The figure shows three views and two pictorial views of one solid part (mm, origin at its lowest corner). Answer the questions. Give positions to 0.01 mm unless a question says otherwise; leave off trailing zeros. Loops run counter-clockwise (first coordinate to the right, second up) from the corner with the lowest first, then second, coordinate; pieces in that order, holes last. Notation, with made-up numbers: (37, 37.5) -> (77, 37.5) arc R24 cw to (77, 51.5) -> close; hole circle Ø5 at (36, -17). An arc over 180 degrees is marked (long way). Answer as CSV lines item,"result". Start each with the question number.
1. Find section C-C, the plane y = 81. Give the vertices of the cut face in (x, z), and give its area (3 significant figures).
2. Flat-ended cylindrical pins translate along their axes: pin 1 Ø3.5 at (x, y) = (11, 152) entering from -Z; pin 2 Ø0.9 at (x, z) = (79.5, 5) entering from +Y; pin 3 Ø1.5 at (x, z) = (80, 5) entering from -Y. Find the tip coordinate at first contact, or state that the pin passes through.
3. Find the intervals of material crossed by line 1 along X through (y, z) = (72, 12.5); line 2 along Y through (x, z) = (29, 8.5); line 3 along Y through (x, z) = (72.5, 6.5), in increasing order.
4. Find section A-A, the plane x = 71. Give the vertices of the cut face in (y, z).
5. Find section B-B, the plane y = 13. Give the vertices of the cut face in (x, z).
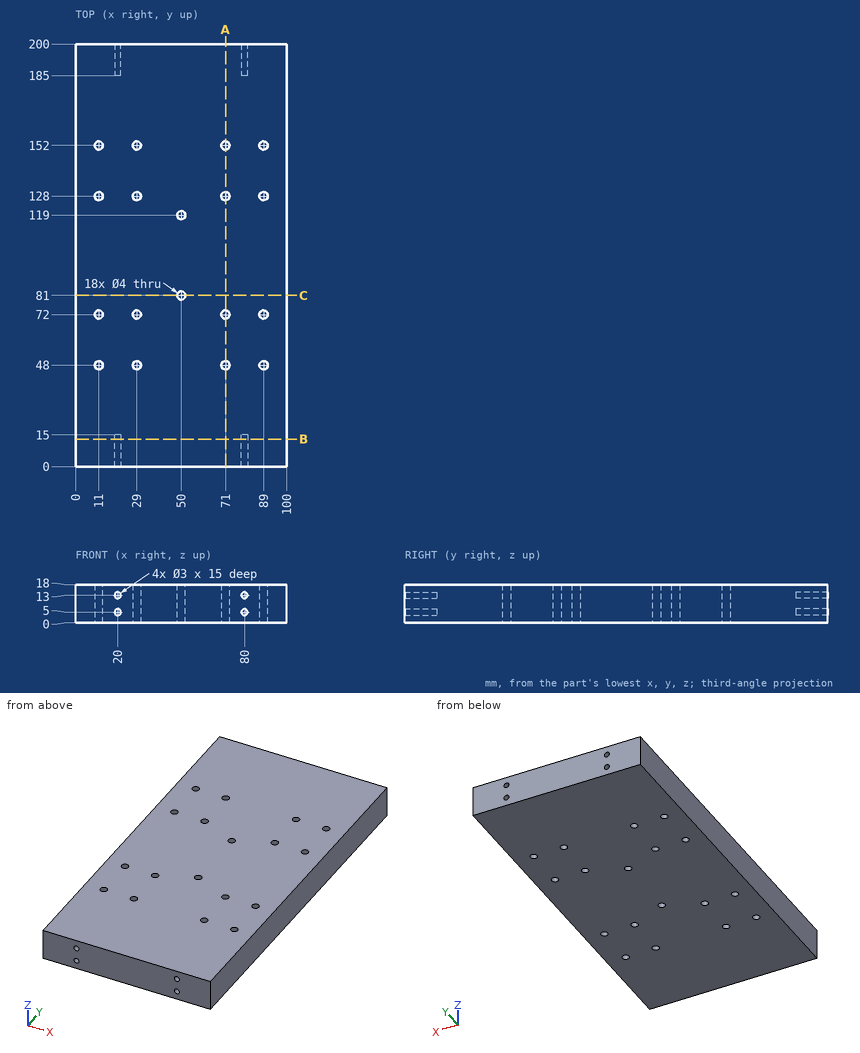
Resolved:
1,outline,"(0, 0) -> (48, 0) -> (48, 18) -> (0, 18) -> close; (52, 0) -> (100, 0) -> (100, 18) -> (52, 18) -> close"
1,area,"1,730 mm^2"
2,pin 1,"passes through"
2,pin 2,"stops at y = 185"
2,pin 3,"stops at y = 15"
3,line 1,"x = 0 to 9, 13 to 27, 31 to 69, 73 to 87, 91 to 100"
3,line 2,"y = 0 to 46, 50 to 70, 74 to 126, 130 to 150, 154 to 200"
3,line 3,"y = 0 to 46.68, 49.32 to 70.68, 73.32 to 126.68, 129.32 to 150.68, 153.32 to 200"
4,outline,"(0, 0) -> (46, 0) -> (46, 18) -> (0, 18) -> close; (50, 0) -> (70, 0) -> (70, 18) -> (50, 18) -> close; (74, 0) -> (126, 0) -> (126, 18) -> (74, 18) -> close; (130, 0) -> (150, 0) -> (150, 18) -> (130, 18) -> close; (154, 0) -> (200, 0) -> (200, 18) -> (154, 18) -> close"
5,outline,"(0, 0) -> (100, 0) -> (100, 18) -> (0, 18) -> close; hole circle Ø3 at (20, 5); hole circle Ø3 at (20, 13); hole circle Ø3 at (80, 5); hole circle Ø3 at (80, 13)"
